from build123d import *

# Parameters (mm, degrees)
CROQUIS1_R              = 2
SALIENTE_EXTRUIR1_DEPTH = 4


with BuildPart() as part:
    # Croquis1 → Saliente-Extruir1 (new body)
    with BuildSketch(Plane.XY):
        Polygon((37.5, 12.25), (-37.5, 12.25), (-37.5, 4), (-33.5, 4), (-33.5, -4), (-37.5, -4), (-37.5, -12.25), (-7, -12.25), (-7, -16.25), (7, -16.25), (7, -12.25), (37.5, -12.25), (37.5, -4), (33.5, -4), (33.5, 4), (37.5, 4), align=None)
        Circle(CROQUIS1_R, mode=Mode.SUBTRACT)
    extrude(amount=SALIENTE_EXTRUIR1_DEPTH)


solid = part.part
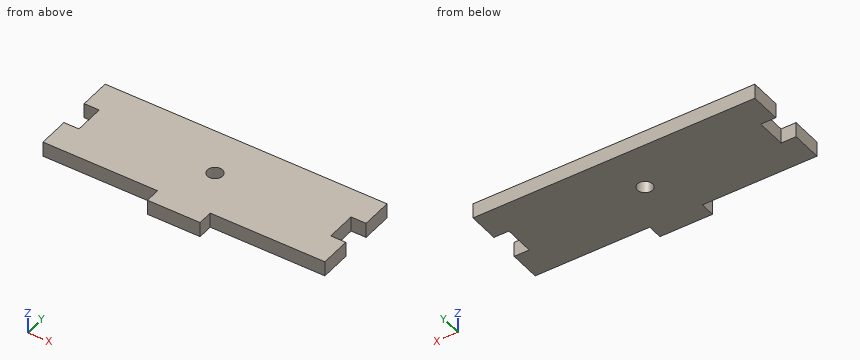
For this review, take the finished solid that the model builds, in its own axes (mm). Give positions to 0.01 mm unless a question says otherwise; leave off trailing zeros. Loops run counter-clockwise (first coordinate to the right, second up) from the corner with the lowest first, then second, coordinate; pieces in that order, holes last. Notation, with made-up numbers: (78, 85.25) - (84, 85.25) arc R15 cw to (84, 111.25) - close; hole circle Ø2 at (-25.5, 76). An arc over 180 degrees is marked (long way). Write each question's results on one line, items separated by ' | '.
(1) Take a section at A-A (x = 0). Give the boundary of the cut face in (y, z).
Conclusion:
outline: (-16.25, 0) - (-2, 0) - (-2, 4) - (-16.25, 4) - close; (2, 0) - (12.25, 0) - (12.25, 4) - (2, 4) - close
(2) For pin 1 Ø2 at (y, z) = (-0.5, 2.5) entering from -X; pin 2 Ø2 at (x, z) = (-20.5, 2) entering from -Y; pin 3 Ø2 at (y, z) = (-13.5, 2) entering from -X, all flat-tipped, find the tip position at first contact; note any pin that passes through.
Conclusion:
pin 1: x = -33.5 | pin 2: y = -12.25 | pin 3: x = -7
(3) Take a section at B-B (y = 0). Give the boundary of the cut face in (x, z), then the cut area to 3 significant figures.
Conclusion:
outline: (-33.5, 0) - (-2, 0) - (-2, 4) - (-33.5, 4) - close; (2, 0) - (33.5, 0) - (33.5, 4) - (2, 4) - close | area: 252 mm^2
(4) For line 1 along Y through (x, z) = (0, 2.95); line 2 along Y through (x, z) = (-34, 1.95); line 3 along X through (y, z) = (-14, 1.4), list the stretches that pass through material, from the lowest coordinate up.
Conclusion:
line 1: -16.25 to -2, 2 to 12.25 | line 2: -12.25 to -4, 4 to 12.25 | line 3: -7 to 7
(5) Take a section at D-D (y = -14). Give the boundary of the cut face in (x, z), then the cut area to 3 significant figures.
Conclusion:
outline: (-7, 0) - (7, 0) - (7, 4) - (-7, 4) - close | area: 56.0 mm^2
(6) Take a section at C-C (z = 2.6). Give the boundary of the cut face in (x, y), then the cut area to 3 significant figures.
Conclusion:
outline: (-37.5, -12.25) - (-7, -12.25) - (-7, -16.25) - (7, -16.25) - (7, -12.25) - (37.5, -12.25) - (37.5, -4) - (33.5, -4) - (33.5, 4) - (37.5, 4) - (37.5, 12.25) - (-37.5, 12.25) - (-37.5, 4) - (-33.5, 4) - (-33.5, -4) - (-37.5, -4) - close; hole circle Ø4 at (0, 0) | area: 1,820 mm^2
